from build123d import *

# Parameters (mm, degrees)
SKETCH1_W           = 68
SKETCH1_H           = 32
BOSS_EXTRUDE1_DEPTH = 13
SKETCH2_R           = 1.5
CUT_EXTRUDE1_DEPTH  = 40.761790704
CUT_EXTRUDE2_DEPTH  = 40.761790704
CUT_EXTRUDE3_START  = -34
CUT_EXTRUDE3_DEPTH  = 3
CUT_EXTRUDE4_START  = 31
CUT_EXTRUDE4_DEPTH  = 3
CUT_EXTRUDE5_DEPTH  = 23
CUT_EXTRUDE6_START  = -23
CUT_EXTRUDE6_DEPTH  = 23
FILLET1_R           = 0.5


with BuildPart() as part:
    # Sketch1 → Boss-Extrude1 (new body)
    with BuildSketch(Plane(origin=(0, 0, 0), x_dir=(1, 0, 0), z_dir=(0, 1, 0))):
        Rectangle(SKETCH1_W, SKETCH1_H)
    extrude(amount=BOSS_EXTRUDE1_DEPTH)

    # Sketch2 → Cut-Extrude1 (cut, through all)
    with BuildSketch(Plane(origin=(0, 13, 0), x_dir=(1, 0, 0), z_dir=(0, 1, 0))):
        with Locations(Location((-28, 7.5, 0), (0, 0, 270))):
            Circle(SKETCH2_R)
        with Locations(Location((-28, -7.5, 0), (0, 0, 270))):
            Circle(SKETCH2_R)
        with Locations(Location((28, -7.5, 0), (0, 0, 270))):
            Circle(SKETCH2_R)
        with Locations(Location((28, 7.5, 0), (0, 0, 270))):
            Circle(SKETCH2_R)
        with Locations(Location((-22.5, 13, 0), (0, 0, 270))):
            Circle(SKETCH2_R)
        with Locations(Location((-7.5, 13, 0), (0, 0, 270))):
            Circle(SKETCH2_R)
        with Locations(Location((7.5, 13, 0), (0, 0, 270))):
            Circle(SKETCH2_R)
        with Locations(Location((22.5, 13, 0), (0, 0, 270))):
            Circle(SKETCH2_R)
        with Locations(Location((-22.5, -13, 0), (0, 0, 270))):
            Circle(SKETCH2_R)
        with Locations(Location((-7.5, -13, 0), (0, 0, 270))):
            Circle(SKETCH2_R)
        with Locations(Location((7.5, -13, 0), (0, 0, 270))):
            Circle(SKETCH2_R)
        with Locations(Location((22.5, -13, 0), (0, 0, 270))):
            Circle(SKETCH2_R)
    extrude(amount=-CUT_EXTRUDE1_DEPTH, mode=Mode.SUBTRACT)

    # Sketch3 → Cut-Extrude2 (cut, through all)
    with BuildSketch(Plane(origin=(0, 13, 0), x_dir=(1, 0, 0), z_dir=(0, 1, 0))):
        with BuildLine():
            Line((-2.5, -2.5), (-2.5, 2.5))
            ThreePointArc((-2.5, 2.5), (0, 5), (2.5, 2.5))
            Line((2.5, 2.5), (2.5, -2.5))
            ThreePointArc((2.5, -2.5), (0, -5), (-2.5, -2.5))
        make_face()
        with BuildLine():
            Line((-8.5, -3.5), (-8.5, 3.5))
            ThreePointArc((-8.5, 3.5), (-7, 5), (-5.5, 3.5))
            Line((-5.5, 3.5), (-5.5, -3.5))
            ThreePointArc((-5.5, -3.5), (-7, -5), (-8.5, -3.5))
        make_face()
        with BuildLine():
            Line((8.5, -3.5), (8.5, 3.5))
            ThreePointArc((8.5, 3.5), (7, 5), (5.5, 3.5))
            Line((5.5, 3.5), (5.5, -3.5))
            ThreePointArc((5.5, -3.5), (7, -5), (8.5, -3.5))
        make_face()
    extrude(amount=-CUT_EXTRUDE2_DEPTH, mode=Mode.SUBTRACT)

    # Sketch5 → Cut-Extrude3 (cut)
    with BuildSketch(Plane(origin=(0, 0, 0), x_dir=(0, 0, -1), z_dir=(1, 0, 0)).offset(CUT_EXTRUDE3_START)):
        with BuildLine():
            Line((16, 7.41504717), (16, 13))
            Line((16, 13), (-16, 13))
            Line((-16, 13), (-16, 7.41504717))
            ThreePointArc((-16, 7.41504717), (0, 2.5), (16, 7.41504717))
        make_face()
    extrude(amount=CUT_EXTRUDE3_DEPTH, mode=Mode.SUBTRACT)

    # Sketch6 → Cut-Extrude4 (cut)
    with BuildSketch(Plane(origin=(0, 0, 0), x_dir=(0, 0, -1), z_dir=(1, 0, 0)).offset(CUT_EXTRUDE4_START)):
        with BuildLine():
            Line((16, 7.41504717), (16, 13))
            Line((16, 13), (-16, 13))
            Line((-16, 13), (-16, 7.41504717))
            ThreePointArc((-16, 7.41504717), (0, 2.5), (16, 7.41504717))
        make_face()
    extrude(amount=CUT_EXTRUDE4_DEPTH, mode=Mode.SUBTRACT)

    # Sketch7 → Cut-Extrude5 (cut)
    with BuildSketch(Plane.ZY.offset(31)):
        with BuildLine():
            Line((-4, 13), (4, 13))
            Line((4, 13), (4, 10))
            ThreePointArc((4, 10), (3.707106781, 9.292893219), (3, 9))
            Line((3, 9), (-3, 9))
            ThreePointArc((-3, 9), (-3.707106781, 9.292893219), (-4, 10))
            Line((-4, 10), (-4, 13))
        make_face()
    extrude(amount=-CUT_EXTRUDE5_DEPTH, mode=Mode.SUBTRACT)

    # Sketch8 → Cut-Extrude6 (cut)
    with BuildSketch(Plane(origin=(31, 0, 0), x_dir=(0, 0, -1), z_dir=(1, 0, 0)).offset(CUT_EXTRUDE6_START)):
        with BuildLine():
            Line((4, 13), (-4, 13))
            Line((-4, 13), (-4, 10))
            ThreePointArc((-4, 10), (-3.707106781, 9.292893219), (-3, 9))
            Line((-3, 9), (3, 9))
            ThreePointArc((3, 9), (3.707106781, 9.292893219), (4, 10))
            Line((4, 10), (4, 13))
        make_face()
    extrude(amount=CUT_EXTRUDE6_DEPTH, mode=Mode.SUBTRACT)

    # Fillet1
    fillet1_edges = [part.edges().sort_by_distance(p)[0] for p in [
        (-8.414213562, 11.5, -4),
        (-8.414213562, 11.5, 4),
        (-8.5, 9.034074174, 3.258819045),
        (-8.454681198, 9.499830019, 3.865927225),
        (-8.5, 9, 0),
        (-8.454681197, 9.499830019, -3.865927225),
        (-8.5, 9.034074174, -3.258819045),
        (8.414213562, 11.5, -4),
        (8.5, 9.034074174, -3.258819045),
        (8.454681197, 9.499830019, -3.865927225),
        (8.5, 9, 0),
        (8.454681198, 9.499830019, 3.865927225),
        (8.5, 9.034074174, 3.258819045),
        (8.414213562, 11.5, 4),
    ]]
    fillet(fillet1_edges, radius=FILLET1_R)


solid = part.part
The model under review builds one solid part; all positions refer to its coordinate system, in mm. A direction names the side the tool comes from. Coordinates: 2 decimals unless noted, no trailing zeros. Order: outer loops, then holes, each group sorted by start corner. A loop starts at its lowest first (then second) coordinate and runs counter-clockwise, first axis right, second up. Notation, with made-up numbers: (2.25, -19.75) -> (25.25, -19.75) arc R23 cw to (25.25, 13.25) -> close; hole circle Ø1 at (75.5, -39). An arc over 180 degrees is marked (long way). Answer in a Markdown table with one row per item.
(1) Consider section A-A (x = 28). Write out the cut boundary in (y, z).
Answers:
| item | result |
|---|---|
| outline | (0, -16) -> (13, -16) -> (13, -9) -> (0, -9) -> close; (0, -6) -> (13, -6) -> (13, -4) -> (10, -4) arc R1 cw to (9, -3) -> (9, 3) arc R1 cw to (10, 4) -> (13, 4) -> (13, 6) -> (0, 6) -> close; (0, 9) -> (13, 9) -> (13, 16) -> (0, 16) -> close |
(2) The part is to be moulded in two halves that separate along X. For faces 5 (the flat face through (0, 13, -7)), 6 (the cylindrical face through (24, 7, 13)), 7 (the flat face through (31, 8, 0)), say which applies: +X half, -X half, draft (parallel to the pull), parting line (faces both ways), or undercut.
Answers:
| item | result |
|---|---|
| face 5 | draft |
| face 6 | undercut |
| face 7 | +X half |
(3) Consider section D-D (x = -11.5). Write out the cut boundary in (y, z).
Answers:
| item | result |
|---|---|
| outline | (0, -16) -> (13, -16) -> (13, -4) -> (10, -4) arc R1 cw to (9, -3) -> (9, 3) arc R1 cw to (10, 4) -> (13, 4) -> (13, 16) -> (0, 16) -> close |
(4) Insertion check: pin 1 (5 mm diameter, centred on x = 24, z = 8.5, fed in from -Y); pin 2 (2 mm diameter, centred on y = 4.5, z = 1, fed in from -X); pin 3 (2.5 mm diameter, centred on x = -7.5, z = 13, fed in from +Y); pin 4 (5.5 mm diameter, centred on y = 5.5, z = -1.5, fed in from +X). Each pin has a flat end and moves straight along its axis. Give the tip position at first contact, or say it passes through.
Answers:
| item | result |
|---|---|
| pin 1 | y = 0 |
| pin 2 | x = -31 |
| pin 3 | through |
| pin 4 | x = 31 |
(5) Consider section C-C (z = 7.5). Write out the cut boundary in (x, y), plus the area to 3 significant figures.
Answers:
| item | result |
|---|---|
| outline | (-34, 0) -> (-29.5, 0) -> (-29.5, 13) -> (-31, 13) -> (-31, 3.5) -> (-34, 3.5) -> close; (-26.5, 0) -> (26.5, 0) -> (26.5, 13) -> (-26.5, 13) -> close; (29.5, 0) -> (34, 0) -> (34, 3.5) -> (31, 3.5) -> (31, 13) -> (29.5, 13) -> close |
| area | 749 mm² |
(6) Wall thickness on line 1 along X through (y, z) = (3.5, -13); line 2 along X through (y, z) = (4, 7.5); line 3 along X through (y, z) = (3, -4): over which ranges is each line inside the solid? List them lowest first.
Answers:
| item | result |
|---|---|
| line 1 | -34 to -24, -21 to -9, -6 to 6, 9 to 21, 24 to 34 |
| line 2 | -31 to -29.5, -26.5 to 26.5, 29.5 to 31 |
| line 3 | -31 to -8.41, -5.59 to -2, 2 to 5.59, 8.41 to 31 |
(7) Machinability: for faces 1 (the flat face through (0, 0, -7)), 2 (the flat face through (-5.5, 7, 0)), 3 (the cylindrical face through (-32.5, 2.5, 0.2)), 4 (the cylindrical face through (32.5, 2.5, 0.2)), which of the approach directions +Z, -Z, +X, -X, +Y, -Y give a long, thin tool a straight path to every point of the face, cutting with its end or side? Answer none if there is none.
Answers:
| item | result |
|---|---|
| face 1 | +Z, -Z, +X, -X, -Y |
| face 2 | +Y, -Y |
| face 3 | -X, +Y |
| face 4 | +X, +Y |
(8) Consider section B-B (z = 12.5). Write out the cut boundary in (x, y).
Answers:
| item | result |
|---|---|
| outline | (-34, 0) -> (-23.91, 0) -> (-23.91, 13) -> (-31, 13) -> (-31, 5.39) -> (-34, 5.39) -> close; (-21.09, 0) -> (-8.91, 0) -> (-8.91, 13) -> (-21.09, 13) -> close; (-6.09, 0) -> (6.09, 0) -> (6.09, 13) -> (-6.09, 13) -> close; (8.91, 0) -> (21.09, 0) -> (21.09, 13) -> (8.91, 13) -> close; (23.91, 0) -> (34, 0) -> (34, 5.39) -> (31, 5.39) -> (31, 13) -> (23.91, 13) -> close |
